Check sheet for the drawn part. Datum: minimum x, y, z corner. Units: mm. A direction names the side the tool comes from. Give positions to 0.01 mm unless a question says otherwise; leave off trailing zeros. Order: outer loops, then holes, each group sorted by start corner. A loop starts at its lowest first (then second) coordinate and runs counter-clockwise, first axis right, second up. Notation, with made-up numbers: M -11,40 L 27,40 A27 ccw 27,60 Z; hole C -25.75,-30.75 d2. An arc over 180 degrees is marked long. Put each result on its own line as item: value. Start each with the question number.
Q1. Material ranges on L1, parallel to Z at x = 9, y = 5.75; L2, parallel to Y at x = 5, z = 4.25; L3, parallel to Z at x = 4.25, y = 5.5, recorded low to high.
Q2. Section check A-A on z = 10.25. Record the cut outline in (x, y).
Q3. Section check B-B on x = 5. Record the cut outline in (y, z).
Q4. Section check C-C on z = 4. Record the cut outline in (x, y), then the cut area to 3 significant figures.
Q5. Go/stop test with flat-tipped pins: pin 1 (1.5 mm diameter, centred on y = 5, z = 3.5, fed in from +X); pin 2 (4 mm diameter, centred on x = 8, z = 3.5, fed in from -Y); pin 3 (1.5 mm diameter, centred on x = 7.5, y = 1, fed in from -Z). Record where each tip stops, or that it passes through.
Q6. Section check D-D on z = 6.25. Record the cut outline in (x, y).
Q7. Mould release check, pull along Y, two halves, no side actions. Record for the marked faces 4, 5 and 6: +Y half, -Y half, draft (parallel to the pull), parting line (faces both ways), or undercut.
Q8. Access from +Z, -Z, +X, -X, +Y, -Y to the whole of each face (thin tool, end or side, straight path). Record for the marked faces 1, 2 and 3.
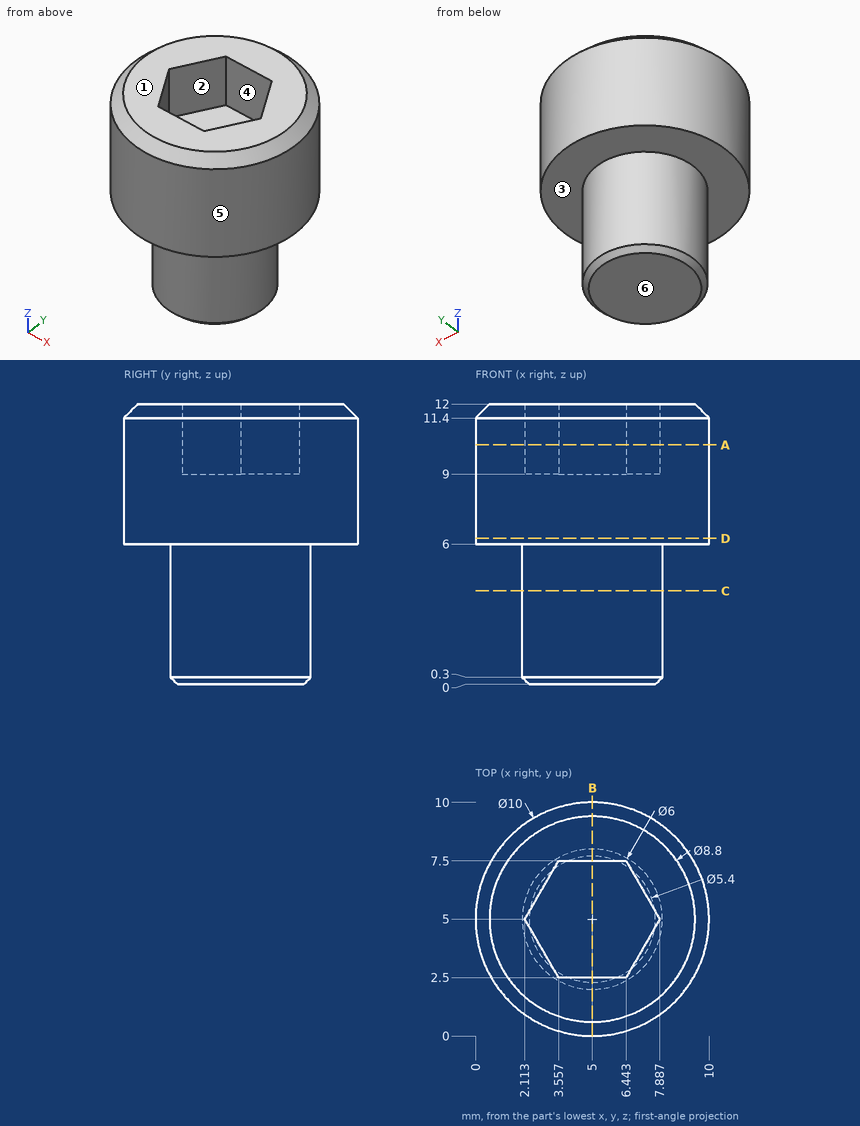
Results found:
1. L1: z = 6 to 12
1. L2: y = 2 to 8
1. L3: z = 0 to 9
2. outline: C 5,5 d10; hole M 2.11,5 L 3.56,2.5 L 6.44,2.5 L 7.89,5 L 6.44,7.5 L 3.56,7.5 Z
3. outline: M 0,6 L 2,6 L 2,0.3 L 2.3,0 L 7.7,0 L 8,0.3 L 8,6 L 10,6 L 10,11.4 L 9.4,12 L 7.5,12 L 7.5,9 L 2.5,9 L 2.5,12 L 0.6,12 L 0,11.4 Z
4. outline: C 5,5 d6
4. area: 28.3 mm^2
5. pin 1: stops at x = 8
5. pin 2: stops at y = 2.17
5. pin 3: stops at z = 6
6. outline: C 5,5 d10
7. face 4: undercut
7. face 5: parting line
7. face 6: draft
8. face 1: +Z, +X, -X, +Y, -Y
8. face 2: +Z
8. face 3: -Z
